Could you check a few things on this model? Use its own coordinates, in mm. A direction names the side the tool comes from. Round coordinates to 2 decimals unless told otherwise and drop trailing zeros. Loops run counter-clockwise (first coordinate to the right, second up) from the corner with the lowest first, then second, coordinate; pieces in that order, holes last.
from build123d import *

# Parameters (mm, degrees)
F0_R     = 2.25
F1_DEPTH = 5
F3_DEPTH = 6
F4_R     = 1.75
F5_DEPTH = 29.243641


with BuildPart() as f1:
    # F0 (on Front) → F1 (new body)
    with BuildSketch(Plane.XZ):
        Polygon((37.5, -3), (37.5, 3), (31.5, 3), align=None)
        Polygon((31.5, 3), (37.5, 3), (19.82233, 20.67767), (16.82233, 17.67767), align=None)
        Polygon((37.5, -3), (31.5, 3), (-37.5, 3), (-37.5, -3), align=None)
        with Locations((-30.5, 0)):
            Circle(F0_R, mode=Mode.SUBTRACT)
        with Locations((30.5, 0)):
            Circle(F0_R, mode=Mode.SUBTRACT)
    extrude(amount=F1_DEPTH)

    # F2 (on face) → F3 (join)
    with BuildSketch(Plane(origin=(0, 0, 0), x_dir=(-1, 0, 0), z_dir=(0, 1, 0))):
        Polygon((-20.357864, 14.142136), (-16.82233, 17.67767), (-19.82233, 20.67767), (-23.357864, 17.142136), align=None)
    extrude(amount=F3_DEPTH)

    # F4 (on face) → F5 (cut, through all)
    with BuildSketch(Plane(origin=(-0.42767, 0, 0.42767), x_dir=(0, -1, 0), z_dir=(-0.707107, 0, 0.707107))):
        with Locations((-3.5, 26.516504)):
            Circle(F4_R)
    extrude(amount=-F5_DEPTH, mode=Mode.SUBTRACT)


solid = f1.part
Item 1: If we section it at B-B, the plane z = 0: Please give me the cut outline in (x, y), then the cut area to 3 significant figures.
Results list:
outline: (-37.5, -5) - (-32.75, -5) - (-32.75, 0) - (-37.5, 0) - close; (-28.25, -5) - (28.25, -5) - (28.25, 0) - (-28.25, 0) - close; (32.75, -5) - (37.5, -5) - (37.5, 0) - (32.75, 0) - close
area: 330 mm2
Item 2: For faces 1 (the cylindrical face through (32.58, -2.46, -0.86)), 2 (the flat face through (-3, -2, 3)), which set-ups out of +Z, -Z, +X, -X, +Y, -Y let a thin tool reach every point of the face, with its end or its side?
Results list:
face 1: +Y, -Y
face 2: -X, +Y, -Y
Item 3: We'd pull the mould along X, two halves only. Please class faces 3 (the flat face through (22.212, 1.625, 15.996)), 4 (the flat face through (-37.5, -2, 0)), 5 (the cylindrical face through (20.12, 5.25, 17.49)): released by +X, released by -X, zero draft, split by the parting line, or undercut.
Results list:
face 3: released by +X
face 4: released by -X
face 5: undercut
Item 4: If we section it at A-A, the plane x = 30.5: Please give me the cut outline in (y, z), then the cut area to 3 significant figures.
Results list:
outline: (-5, -3) - (0, -3) - (0, -2.25) - (-5, -2.25) - close; (-5, 2.25) - (0, 2.25) - (0, 3) - (-5, 3) - close; (-5, 4) - (0, 4) - (0, 10) - (-5, 10) - close
area: 37.5 mm2
Item 5: If we section it at D-D, the plane y = -0.75: Please give me the cut outline in (x, z), then the cut area to 3 significant figures.
Results list:
outline: (-37.5, -3) - (37.5, -3) - (37.5, 3) - (19.82, 20.68) - (16.82, 17.68) - (31.5, 3) - (-37.5, 3) - close; hole circle Ø4.5 at (-30.5, 0); hole circle Ø4.5 at (30.5, 0)
area: 515 mm2
Item 6: Will these pins go through, and if not, where does the flat tip stop? pin 1 (1 mm diameter, centred on y = -1, z = 13, fed in from -X); pin 2 (1.5 mm diameter, centred on x = -1.5, z = 0, fed in from +Y); pin 3 (6 mm diameter, centred on y = -1, z = 17.5, fed in from -X).
Results list:
pin 1: stops at x = 21
pin 2: stops at y = 0
pin 3: stops at x = 16.82
Item 7: If we section it at C-C, the plane x = -30.5: Please give me the cut outline in (y, z), then the cut area to 3 significant figures.
Results list:
outline: (-5, -3) - (0, -3) - (0, -2.25) - (-5, -2.25) - close; (-5, 2.25) - (0, 2.25) - (0, 3) - (-5, 3) - close
area: 7.50 mm2
Item 8: If I drill on line 1 along Z through (x, y) = (30.5, -1.55); line 2 along Z through (x, y) = (-30.5, -2.75); line 3 along Y through (x, z) = (-14, 0), over which ranges is the centre line in solid material (lowest first)?
Results list:
line 1: z = -3 to -2.25, 2.25 to 3, 4 to 10
line 2: z = -3 to -2.25, 2.25 to 3
line 3: y = -5 to 0
